```python
from build123d import *

# Parameters (mm, degrees)
BOSS_EXTRUDE1_DEPTH = 40
FILLET1_R           = 3
SKETCH2_W           = 25
SKETCH2_H           = 11
CUT_EXTRUDE1_DEPTH  = 158.48015748
SKETCH3_W           = 20
SKETCH3_H           = 49
CUT_EXTRUDE2_DEPTH  = 170.705627485


with BuildPart() as part:
    # Sketch1 → Boss-Extrude1 (new body)
    with BuildSketch(Plane.XY):
        Polygon((0, 0), (0, 160), (20, 160), (20, 20), (60, 20), (60, 0), align=None)
    extrude(amount=BOSS_EXTRUDE1_DEPTH)

    # Fillet1
    fillet1_edges = [part.edges().sort_by_distance(p)[0] for p in [
        (60, 10, 40),
        (60, 10, 0),
    ]]
    fillet(fillet1_edges, radius=FILLET1_R)

    # Sketch2 → Cut-Extrude1 (cut, through all)
    with BuildSketch(Plane(origin=(0, 20, 0), x_dir=(1, 0, 0), z_dir=(0, 1, 0))):
        with Locations((37.5, -20)):
            Rectangle(SKETCH2_W, SKETCH2_H)
    extrude(amount=-CUT_EXTRUDE1_DEPTH, mode=Mode.SUBTRACT)

    # Sketch3 → Cut-Extrude2 (cut, through all)
    with BuildSketch(Plane(origin=(20, 0, 0), x_dir=(0, 0, -1), z_dir=(1, 0, 0))):
        with Locations((-20, 99.5)):
            Rectangle(SKETCH3_W, SKETCH3_H)
    extrude(amount=-CUT_EXTRUDE2_DEPTH, mode=Mode.SUBTRACT)


solid = part.part
```
Verification items for the finished model (mm, model axes). A direction names the side the tool comes from. Give positions to 0.01 mm unless a question says otherwise; leave off trailing zeros. Order: outer loops, then holes, each group sorted by start corner. A loop starts at its lowest first (then second) coordinate and runs counter-clockwise, first axis right, second up. Notation, with made-up numbers: (27.5, 6.25) -> (81.5, 6.25) arc R20 ccw to (81.5, 23.25) -> close; hole circle Ø11 at (88, 8.25). An arc over 180 degrees is marked (long way). One line per item, written item: value.
(1) Sectioned sample at B-B on x = 44. Record the cut outline in (y, z).
Final values:
outline: (0, 0) -> (20, 0) -> (20, 14.5) -> (0, 14.5) -> close; (0, 25.5) -> (20, 25.5) -> (20, 40) -> (0, 40) -> close
(2) Draft check along Y on faces 1 (the face through (10, 160, 20)), 2 (the face through (10, 75, 20)), 3 (the face through (50, 10, 20)). Enter one of: pulls with the +Y half, pulls with the -Y half, needs draft (parallel to the pull), parting line crosses it, or undercut.
Final values:
face 1: pulls with the +Y half
face 2: undercut
face 3: needs draft
(3) Gauge pin test, flat ends, axial feed: pin 1 (6 mm diameter, centred on y = 116.5, z = 32, fed in from +X); pin 2 (20 mm diameter, centred on x = 45, z = 19, fed in from +Y); pin 3 (12 mm diameter, centred on y = 13.5, z = 18.5, fed in from -X). Record the tip position at first contact, or that the pin passes through.
Final values:
pin 1: x = 20
pin 2: y = 20
pin 3: x = 0
(4) Sectioned sample at A-A on y = 109.5. Record the cut outline in (x, z), then the cut area to 3 significant figures.
Final values:
outline: (0, 0) -> (20, 0) -> (20, 10) -> (0, 10) -> close; (0, 30) -> (20, 30) -> (20, 40) -> (0, 40) -> close
area: 400 mm^2
(5) Sectioned sample at C-C on z = 17. Record the cut outline in (x, y).
Final values:
outline: (0, 0) -> (25, 0) -> (25, 20) -> (20, 20) -> (20, 75) -> (0, 75) -> close; (0, 124) -> (20, 124) -> (20, 160) -> (0, 160) -> close; (50, 0) -> (60, 0) -> (60, 20) -> (50, 20) -> close
(6) Tool access check on faces 4 (the face through (40, 20, 11)), 5 (the face through (0, 61, 20)), 6 (the face through (10, 99, 10)), 7 (the face through (25, 10, 20)), 8 (the face through (16, 63, 0)). Record the directions out of +Z, -Z, +X, -X, +Y, -Y that give a thin tool (end or side, any length) a straight path to the whole face; none if there is none.
Final values:
face 4: +Z, -Z, +X, +Y
face 5: +Z, -Z, -X, +Y, -Y
face 6: +X, -X
face 7: +Y, -Y
face 8: -Z, +X, -X, +Y, -Y
(7) Scan lines: line 1 along Y through (x, z) = (12, 27); line 2 along Z through (x, y) = (19.5, 118.5); line 3 along Y through (x, z) = (40.5, 35.5). Record each from-to range of solid material in increasing order. Write a range as [from, to].
Final values:
line 1: [0, 75], [124, 160]
line 2: [0, 10], [30, 40]
line 3: [0, 20]
(8) Sectioned sample at D-D on z = 27.5. Record the cut outline in (x, y), then the cut area to 3 significant figures.
Final values:
outline: (0, 0) -> (60, 0) -> (60, 20) -> (20, 20) -> (20, 75) -> (0, 75) -> close; (0, 124) -> (20, 124) -> (20, 160) -> (0, 160) -> close
area: 3,020 mm^2
